Here's how the part is built. I have some questions about the finished solid (model axes, mm). Face numbers are marked on the shaded views. A direction names the side the tool comes from. Coordinates: 2 decimals unless noted, no trailing zeros. Order: outer loops, then holes, each group sorted by start corner. A loop starts at its lowest first (then second) coordinate and runs counter-clockwise, first axis right, second up. Notation, with made-up numbers: (-7.75, -29) - (41.25, -29) arc R5 cw to (41.25, -21) - close; hole circle Ø8 at (-11.75, -34). An arc over 180 degrees is marked (long way). Answer in a Markdown table with one row per item. Add a question column.
Item 1: Will these pins go through, and if not, where does the flat tip stop? pin 1 Ø12 at (x, z) = (-14.5, -8.5) entering from +Y; pin 2 Ø1.6 at (x, y) = (-87.5, 51.5) entering from -Z; pin 3 Ø1.5 at (y, z) = (56.5, -6) entering from -X.
Item 2: I want a section at B-B (y = 27). Please give me the cut outline in (x, z).
Item 3: If I drill on line 1 along X through (y, z) = (50.8, -1.7); line 2 along Y through (x, z) = (-87.3, -2.85); line 3 along Y through (x, z) = (-54.5, -17.5), over which ranges is the centre line in solid material (lowest first)? Write a range as from..to.
Item 4: I want a section at C-C (z = -14). Please give me the cut outline in (x, y), plus the area to 3 significant figures.
Item 5: On a 3-axis mill with a long thin cutter (end or side, diameter ignored), from which of +Z, -Z, +X, -X, +Y, -Y can I reach the whole of each face in a straight line? I mean the marked faces 1, 2 and 3. Say none if no direction works.
Item 6: I want a section at A-A (x = 49). Please give me the cut outline in (y, z).
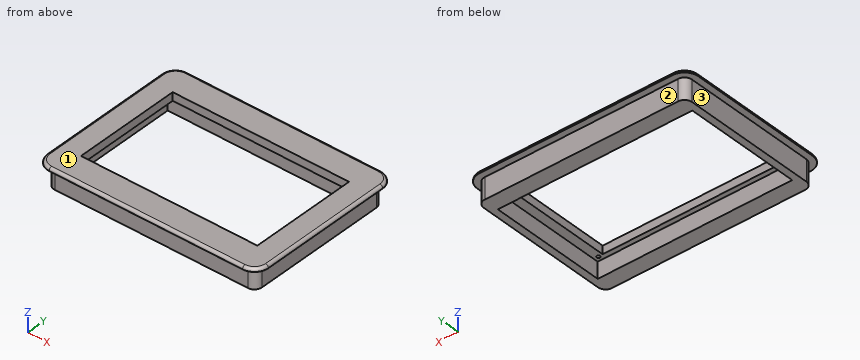
```python
from build123d import *

# Parameters (mm, degrees)
PAD001_DEPTH    = 3
PAD002_DEPTH    = 20
FILLET_R        = 2.5
SKETCH005_W     = 166
SKETCH005_H     = 101
POCKET001_DEPTH = 23.001
SKETCH006_W     = 183
SKETCH006_H     = 110
POCKET002_DEPTH = 15.3
SKETCH007_R     = 1.6
POCKET003_DEPTH = 5


with BuildPart() as part:
    # Sketch002 → Pad001 (new body)
    with BuildSketch(Plane.XY):
        with BuildLine():
            Line((-91, 76), (91, 76))
            ThreePointArc((104, 63), (100.192388, 72.192388), (91, 76))
            Line((104, 63), (104, -63))
            ThreePointArc((91, -76), (100.192388, -72.192388), (104, -63))
            Line((91, -76), (-91, -76))
            ThreePointArc((-104, -63), (-100.192388, -72.192388), (-91, -76))
            Line((-104, -63), (-104, 63))
            ThreePointArc((-91, 76), (-100.192388, 72.192388), (-104, 63))
        make_face()
    extrude(amount=PAD001_DEPTH)

    # Sketch004 → Pad002 (join)
    with BuildSketch(Plane.XY):
        with BuildLine():
            Line((-91, 70), (91, 70))
            ThreePointArc((98, 63), (95.949747, 67.949747), (91, 70))
            Line((98, 63), (98, -63))
            ThreePointArc((91, -70), (95.949747, -67.949747), (98, -63))
            Line((91, -70), (-91, -70))
            ThreePointArc((-98, -63), (-95.949747, -67.949747), (-91, -70))
            Line((-98, -63), (-98, 63))
            ThreePointArc((-91, 70), (-95.949747, 67.949747), (-98, 63))
        make_face()
    extrude(amount=-PAD002_DEPTH)

    # Fillet
    fillet_edges = [part.edges().sort_by_distance(p)[0] for p in [
        (-104, 0, 3),
        (-100.192388, 72.192388, 3),
        (0, 76, 3),
        (100.192388, 72.192388, 3),
        (104, 0, 3),
        (100.192388, -72.192388, 3),
        (0, -76, 3),
        (-100.192388, -72.192388, 3),
    ]]
    fillet(fillet_edges, radius=FILLET_R)

    # Sketch005 (on Face19 of Pad002) → Pocket001 (cut, through all)
    with BuildSketch(Plane(origin=(0, 0, -20), x_dir=(1, 0, 0), z_dir=(0, 0, -1))):
        Rectangle(SKETCH005_W, SKETCH005_H)
    extrude(amount=-POCKET001_DEPTH, mode=Mode.SUBTRACT)

    # Sketch006 (on Face31 of Pocket001) → Pocket002 (cut)
    with BuildSketch(Plane(origin=(0, 0, -20), x_dir=(1, 0, 0), z_dir=(0, 0, -1))):
        Rectangle(SKETCH006_W, SKETCH006_H)
    extrude(amount=-POCKET002_DEPTH, mode=Mode.SUBTRACT)

    # Sketch007 (on Face32 of Pocket002) → Pocket003 (cut)
    with BuildSketch(Plane(origin=(0, 0, -4.7), x_dir=(1, 0, 0), z_dir=(0, 0, -1))):
        with Locations((-87.3, 50.8)):
            Circle(SKETCH007_R)
        with Locations((87.3, 50.8)):
            Circle(SKETCH007_R)
        with Locations((87.3, -50.8)):
            Circle(SKETCH007_R)
        with Locations((-87.3, -50.8)):
            Circle(SKETCH007_R)
    extrude(amount=-POCKET003_DEPTH, mode=Mode.SUBTRACT)


solid = part.part
```
Values follow:
| question | item | result |
|---|---|---|
| 1 | pin 1 | stops at y = 70 |
| 1 | pin 2 | stops at z = 0.3 |
| 1 | pin 3 | stops at x = -98 |
| 2 | outline | (-104, 0) - (-98, 0) - (-98, -20) - (-91.5, -20) - (-91.5, -4.7) - (-83, -4.7) - (-83, 3) - (-101.5, 3) arc R2.5 ccw to (-104, 0.5) - close; (83, -4.7) - (91.5, -4.7) - (91.5, -20) - (98, -20) - (98, 0) - (104, 0) - (104, 0.5) arc R2.5 ccw to (101.5, 3) - (83, 3) - close |
| 3 | line 1 | x = -98..-88.9, -85.7..85.7, 88.9..98 |
| 3 | line 2 | y = -70..-52.4, -49.2..49.2, 52.4..70 |
| 3 | line 3 | y = -70..-55, 55..70 |
| 4 | outline | (-98, -63) arc R7 ccw to (-91, -70) - (91, -70) arc R7 ccw to (98, -63) - (98, 63) arc R7 ccw to (91, 70) - (-91, 70) arc R7 ccw to (-98, 63) - close; hole (-91.5, -55) - (91.5, -55) - (91.5, 55) - (-91.5, 55) - close |
| 4 | area | 7,270 mm^2 |
| 5 | face 1 | +Z, +X, -X, +Y, -Y |
| 5 | face 2 | -Z, +X, -X, +Y |
| 5 | face 3 | -Z, -X, +Y, -Y |
| 6 | outline | (-76, 0) - (-70, 0) - (-70, -20) - (-55, -20) - (-55, -4.7) - (-50.5, -4.7) - (-50.5, 3) - (-73.5, 3) arc R2.5 ccw to (-76, 0.5) - close; (50.5, -4.7) - (55, -4.7) - (55, -20) - (70, -20) - (70, 0) - (76, 0) - (76, 0.5) arc R2.5 ccw to (73.5, 3) - (50.5, 3) - close |
